from build123d import *

# Parameters (mm, degrees)
F0_W     = 27.6901638135
F0_H     = 18.3629523963
F1_DEPTH = 36.068
F2_R     = 7.4938109385
F2_R_2   = 7.4938128
F3_DEPTH = 57.404
F4_W     = 20.1118043624
F4_H     = 29.0018040687
F5_DEPTH = 0.762
F6_SIZE  = 27.94


with BuildPart() as f1:
    # F0 (on Right) → F1 (new body)
    with BuildSketch(Plane.YZ):
        Polygon((-35.5600006878, 10.0559014827), (-63.8331216878, 10.0559014827), (-63.8331216878, -15.3440985173), (49.550820142, -15.3440985173), (49.550820142, 10.0559014827), (21.2777052075, 10.0559014827), (6.7039346322, 28.418853879), (6.7039346322, 10.0559014827), (-20.9862291813, 10.0559014827), (-20.9862291813, 28.418853879), align=None)
        with Locations((-7.1411472745, 19.2373776808)):
            Rectangle(F0_W, F0_H)
    extrude(amount=-F1_DEPTH)

    # F2 (on Top) → F3 (cut)
    with BuildSketch(Plane.XY):
        with Locations((-19.2373786122, -48.5306568444)):
            Circle(F2_R)
        with Locations((-19.2373786122, 36.5801639855)):
            Circle(F2_R_2)
    extrude(amount=F3_DEPTH, mode=Mode.SUBTRACT)

    # F4 (on Right) → F5 (cut)
    with BuildSketch(Plane.YZ):
        with Locations((-6.2667217571, 14.5009020343)):
            Rectangle(F4_W, F4_H)
    extrude(amount=-F5_DEPTH, mode=Mode.SUBTRACT)

    # F6
    f6_edges = [f1.edges().sort_by_distance(p)[0] for p in [
        (-0.762, -6.266722, 28.418854),
    ]]
    chamfer(f6_edges, length=F6_SIZE)


solid = f1.part
Part model, mm, in its own coordinate system. A direction names the side the tool comes from. Give positions to 0.01 mm unless a question says otherwise; leave off trailing zeros. Write each loop counter-clockwise with the first axis right and the second up, starting at its lowest first coordinate (ties: lowest second). Pieces come first, ordered by that corner, then holes.
1) Two-plate mould, pull along X, no slides. Class faces 1 (the face through (-22, -17, 28.419)), 2 (the face through (-36.068, -8, 2)), 3 (the face through (-12.315, 33.71, 4.958)), 4 (the face through (-20.862, -55.846, 4.958)): released by +X, released by -X, zero draft, split by the parting line, or undercut.
Resolved:
face 1: zero draft
face 2: released by -X
face 3: undercut
face 4: undercut
2) Pin check, flat tips, straight feed: pin 1 (16.5 mm diameter, centred on x = -20.5, y = 38.5, fed in from +Z); pin 2 (6 mm diameter, centred on x = -7, y = 13, fed in from +Z); pin 3 (0.5 mm diameter, centred on y = -5, z = 0.5, fed in from +X). Stop position of each tip, or through.
Resolved:
pin 1: stops at z = 10.06
pin 2: stops at z = 24.27
pin 3: stops at x = -0.76
3) Cut at D-D on z = 21. Write the cut outline in (x, y), then the cut area to 3 significant figures.
Resolved:
outline: (-36.07, -26.87) - (0, -26.87) - (0, -16.32) - (-21.28, -16.32) - (-21.28, 3.79) - (0, 3.79) - (0, 12.59) - (-36.07, 12.59) - close
area: 995 mm2
4) Which spindle directions (+Z, -Z, +X, -X, +Y, -Y) get a long thin tool onto all of the face, cutting with end or side? Do faces 5 (the face through (-14.536, -6.126, 14.253)), 6 (the face through (-14, -56, 10.056)), 7 (the face through (-14, 29, 10.056)), 8 (the face through (-19, 37, 0)). Say none if no direction does.
Resolved:
face 5: +Z, +X
face 6: +Z, +X, -X, -Y
face 7: +Z, +X, -X, +Y
face 8: +Z
5) Cut at A-A on y = -9. Write the cut outline in (x, z), then the cut area to 3 significant figures.
Resolved:
outline: (-36.07, -15.34) - (0, -15.34) - (0, 0) - (-0.76, 0) - (-0.76, 0.48) - (-28.7, 28.42) - (-36.07, 28.42) - close
area: 1,170 mm2
6) Probe L1, parallel to Y at x = -23.5, z = 9; L2, parallel to Y at x = -17.5, z = 2; L3, parallel to Y at x = -19, z = 19. List the from-to ranges inside material, lowest first.
Resolved:
L1: y = -63.83 to -54.69, -42.37 to 30.42, 42.74 to 49.55
L2: y = -63.83 to -55.82, -41.24 to 29.29, 43.87 to 49.55
L3: y = -28.46 to -16.32, 3.79 to 14.18
7) Cut at B-B on x = -30. Write the cut outline in (y, z), then the cut area to 3 significant figures.
Resolved:
outline: (-63.83, -15.34) - (49.55, -15.34) - (49.55, 10.06) - (21.28, 10.06) - (6.7, 28.42) - (-20.99, 28.42) - (-35.56, 10.06) - (-63.83, 10.06) - close
area: 3,660 mm2
8) Cut at C-C on z = 7. Write the cut outline in (x, y), then the cut area to 3 significant figures.
Resolved:
outline: (-36.07, -63.83) - (0, -63.83) - (0, -16.32) - (-7.28, -16.32) - (-7.28, 3.79) - (0, 3.79) - (0, 49.55) - (-36.07, 49.55) - close; hole circle Ø14.99 at (-19.24, -48.53); hole circle Ø14.99 at (-19.24, 36.58)
area: 3,590 mm2
